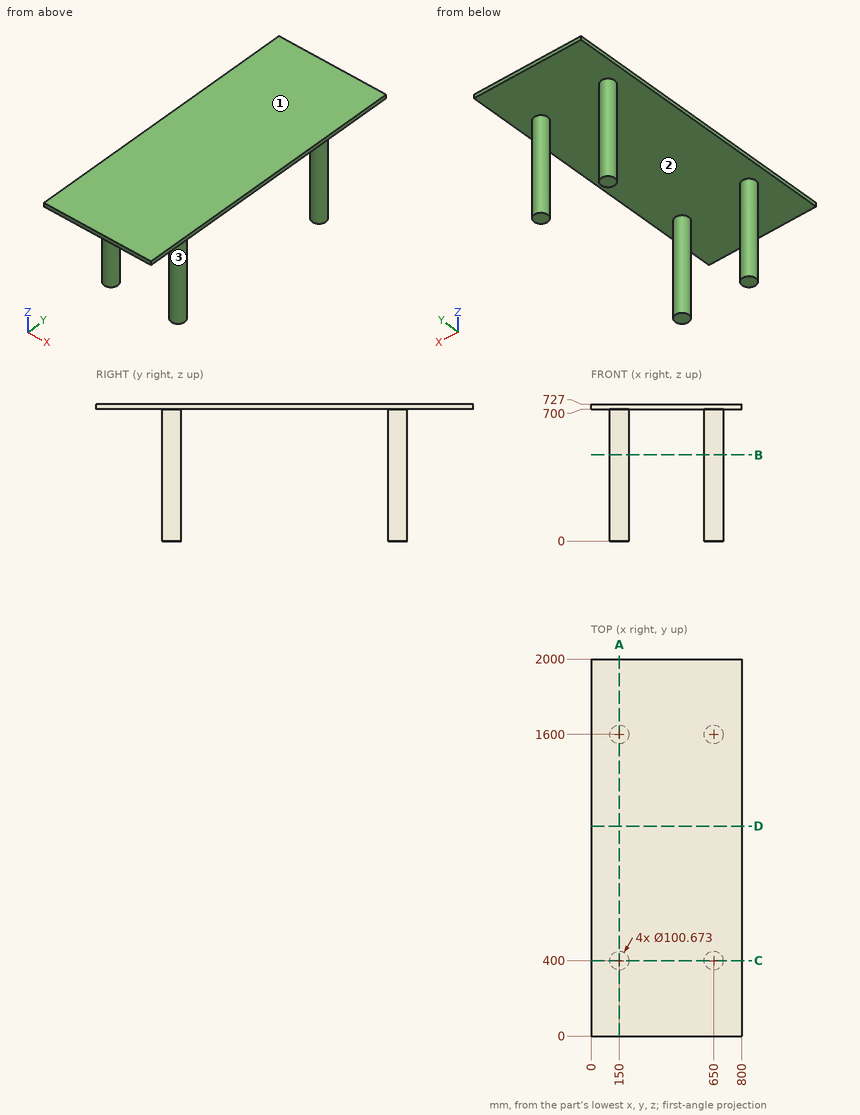
Print and shaded views of the part. All mm, measured from the part's lowest x, y and z. Round coordinates to 2 decimals unless told otherwise and drop trailing zeros. Write each loop counter-clockwise with the first axis right and the second up, starting at its lowest first coordinate (ties: lowest second). Pieces come first, ordered by that corner, then holes.
Item 1: Cut at D-D, the plane y = 1113. Give the cut face in (x, z).
Results:
outline: (0, 700) - (800, 700) - (800, 727) - (0, 727) - close
Item 2: Cut at C-C, the plane y = 400. Give the cut face in (x, z).
Results:
outline: (0, 700) - (99.66, 700) - (99.66, 0) - (200.34, 0) - (200.34, 700) - (599.66, 700) - (599.66, 0) - (700.34, 0) - (700.34, 700) - (800, 700) - (800, 727) - (0, 727) - close
Item 3: Two-plate mould, pull along Y, no slides. Class the marked faces 1, 2 and 3: +Y half, -Y half, draft (parallel to the pull), parting line (faces both ways), or undercut.
Results:
face 1: draft
face 2: undercut
face 3: undercut
Item 4: Cut at B-B, the plane z = 457.5. Give the cut face in (x, y), plus the area to 3 significant figures.
Results:
outline: circle Ø100.67 at (150, 400); circle Ø100.67 at (150, 1600); circle Ø100.67 at (650, 400); circle Ø100.67 at (650, 1600)
area: 31,800 mm2
Item 5: Drop flat-ended pins along their axis: pin 1 Ø10 at (x, z) = (144, 546) entering from -Y; pin 2 Ø1 at (x, y) = (336.5, 918) entering from -Z. Give the stop position or say it passes through.
Results:
pin 1: stops at y = 349.67
pin 2: stops at z = 700
Item 6: Cut at A-A, the plane x = 150. Give the cut face in (y, z).
Results:
outline: (0, 700) - (349.66, 700) - (349.66, 0) - (450.34, 0) - (450.34, 700) - (1549.66, 700) - (1549.66, 0) - (1650.34, 0) - (1650.34, 700) - (2000, 700) - (2000, 727) - (0, 727) - close
Item 7: Probe L1, parallel to Z at x = 544, y = 1776; L2, parallel to X at y = 354.5, z = 633.5; L3, parallel to Y at x = 191, z = 463.5. List the from-to ranges inside material, lowest first.
Results:
L1: z = 700 to 727
L2: x = 128.47 to 171.53, 628.47 to 671.53
L3: y = 370.8 to 429.2, 1570.8 to 1629.2
